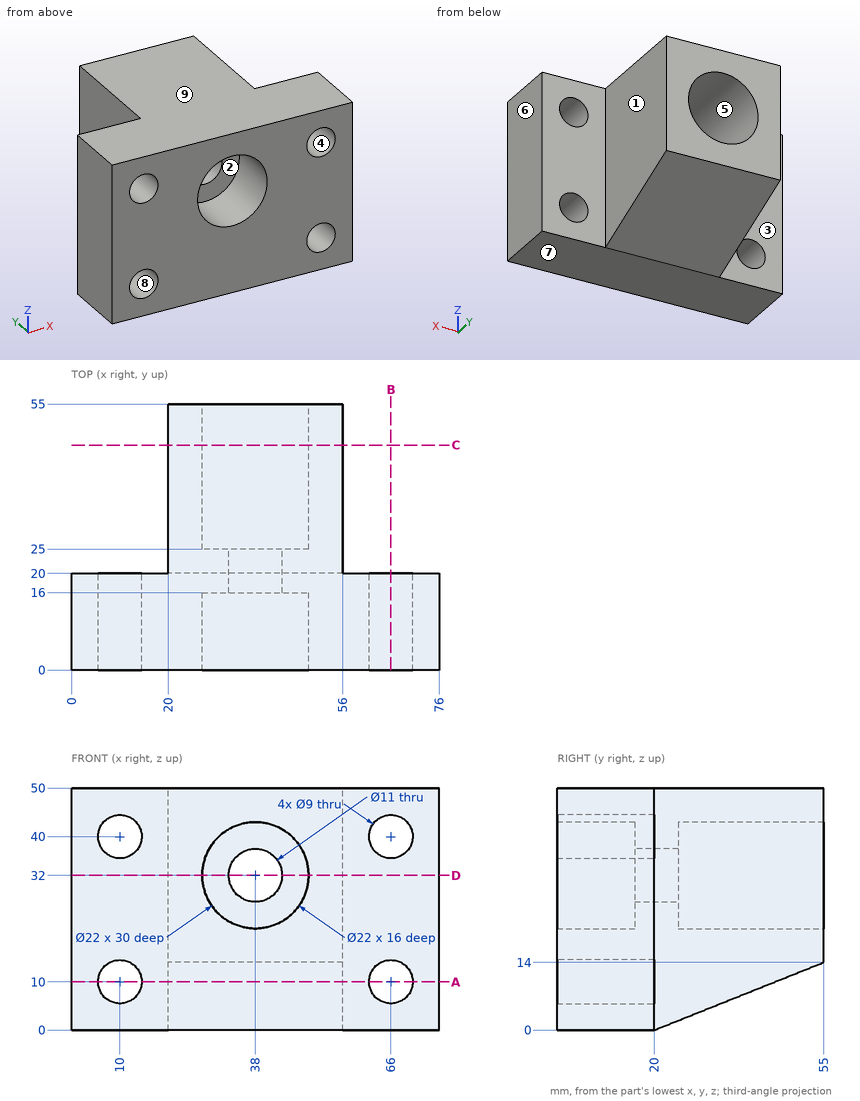
Design review of the part shown in the three views and the two pictorial views. Dimensions are in mm from the part's minimum x, y and z. A direction names the side the tool comes from. Round coordinates to 2 decimals unless told otherwise and drop trailing zeros. Write each loop counter-clockwise with the first axis right and the second up, starting at its lowest first coordinate (ties: lowest second). Pieces come first, ordered by that corner, then holes. Notation, with made-up numbers: (34.5, 14) -> (54.5, 14) arc R30 ccw to (54.5, 37) -> close; hole circle Ø2 at (-17, 89). An arc over 180 degrees is marked (long way). Use one line per item in the form item = value.
1) Take a section at D-D, the plane z = 32. Write out the cut boundary in (x, y), and give its area (3 significant figures).
Found:
outline = (0, 0) -> (27, 0) -> (27, 16) -> (32.5, 16) -> (32.5, 25) -> (27, 25) -> (27, 55) -> (20, 55) -> (20, 20) -> (0, 20) -> close; (43.5, 16) -> (49, 16) -> (49, 0) -> (76, 0) -> (76, 20) -> (56, 20) -> (56, 55) -> (49, 55) -> (49, 25) -> (43.5, 25) -> close
area = 1,670 mm2
2) Clearance check with flat-ended pins moving along their axes: pin 1 (1 mm diameter, centred on x = 13, z = 16, fed in from +Y); pin 2 (10.5 mm diameter, centred on y = 35, z = 26, fed in from -X); pin 3 (10 mm diameter, centred on y = 40, z = 39.5, fed in from +X); pin 4 (8 mm diameter, centred on x = 20.5, z = 32, fed in from -Y). State where each tip first meets the part, or that it passes through.
Found:
pin_1 = 20
pin_2 = 20
pin_3 = 56
pin_4 = 0
3) Take a section at C-C, the plane y = 46.5. Write out the cut boundary in (x, z), and give its area (3 significant figures).
Found:
outline = (20, 10.6) -> (56, 10.6) -> (56, 50) -> (20, 50) -> close; hole circle Ø22 at (38, 32)
area = 1,040 mm2
4) To check wall thickness, follow L1, parallel to X at y = 4.25, z = 40; L2, parallel to Z at x = 6.5, y = 14; L3, parallel to X at y = 31.5, z = 17. State the ranges of each line that lie inside material, in increasing order. Write a range as from..to.
Found:
L1 = 0..5.5, 14.5..30.45, 45.55..61.5, 70.5..76
L2 = 0..7.17, 12.83..37.17, 42.83..50
L3 = 20..56
5) Take a section at A-A, the plane z = 10. Write out the cut boundary in (x, y).
Found:
outline = (0, 0) -> (5.5, 0) -> (5.5, 20) -> (0, 20) -> close; (14.5, 0) -> (61.5, 0) -> (61.5, 20) -> (56, 20) -> (56, 45) -> (20, 45) -> (20, 20) -> (14.5, 20) -> close; (70.5, 0) -> (76, 0) -> (76, 20) -> (70.5, 20) -> close
6) Tool access review of the marked faces 1, 2, 3, 4 and 5: name each direction out of +Z, -Z, +X, -X, +Y, -Y from which nothing blocks a thin tool from reaching the whole face with its end or side.
Found:
face_1 = +Z, -Z, +X, +Y
face_2 = -Y
face_3 = +Z, -Z, -X, +Y
face_4 = +Y, -Y
face_5 = +Y
7) Mouldability with a two-part tool opening along Z and no side actions: class the marked faces 6, 7, 8 and 9 as +Z half, -Z half, draft (parallel to the pull), parting line (faces both ways), or undercut.
Found:
face_6 = draft
face_7 = -Z half
face_8 = undercut
face_9 = +Z half
8) Take a section at B-B, the plane x = 66. Write out the cut boundary in (y, z).
Found:
outline = (0, 0) -> (20, 0) -> (20, 5.5) -> (0, 5.5) -> close; (0, 14.5) -> (20, 14.5) -> (20, 35.5) -> (0, 35.5) -> close; (0, 44.5) -> (20, 44.5) -> (20, 50) -> (0, 50) -> close
